Work out the finished part from the listing and answer in its coordinate system (mm). Face numbers are marked on the shaded views. A direction names the side the tool comes from. Give positions to 0.01 mm unless a question says otherwise; leave off trailing zeros. Loops run counter-clockwise (first coordinate to the right, second up) from the corner with the lowest first, then second, coordinate; pieces in that order, holes last. Notation, with made-up numbers: M -24,77.25 L 25,77.25 A23 cw 25,97.25 Z; hole C 72.5,45 d4. An arc over 180 degrees is marked long. Use a Markdown table: item, result.
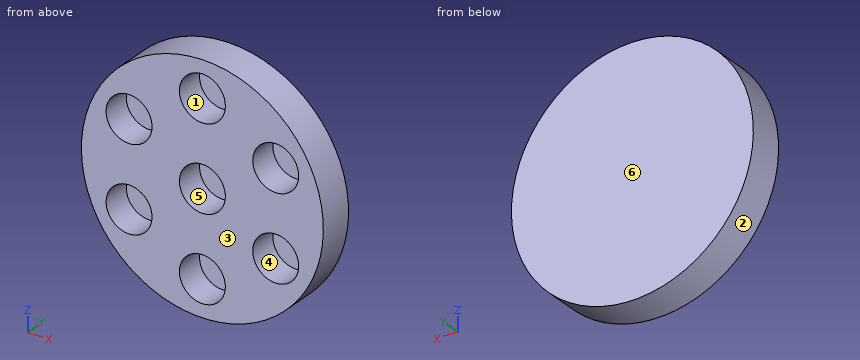
```python
from build123d import *

# Parameters (mm, degrees)
SKETCH1_R           = 25.4
BOSS_EXTRUDE2_DEPTH = 7.62
SKETCH4_R           = 4.826
CUT_EXTRUDE2_DEPTH  = 6.096
CIRPATTERN1_COUNT   = 6
SKETCH5_R           = 4.826
CUT_EXTRUDE6_DEPTH  = 6.096
SCALE1_SCALE        = 0.5


with BuildPart() as part:
    # Sketch1 → Boss-Extrude2 (new body)
    with BuildSketch(Plane(origin=(0, 0, 0), x_dir=(1, 0, 0), z_dir=(0, 1, 0))):
        with Locations(Location((0, 0, 0), (0, 0, 270))):
            Circle(SKETCH1_R)
    extrude(amount=BOSS_EXTRUDE2_DEPTH)

    # Sketch4 → Cut-Extrude2 (cut)
    with BuildSketch(Plane(origin=(0, 0, 0), x_dir=(1, 0, 0), z_dir=(0, 1, 0))):
        with Locations(Location((0, 17.78, 0), (0, 0, 90))):
            Circle(SKETCH4_R)
    cut_extrude2 = extrude(amount=CUT_EXTRUDE2_DEPTH, mode=Mode.SUBTRACT)

    # CirPattern1: Cut-Extrude2 ×6 about axis
    cirpattern1_axis = Axis((0, 0, 0), (0, 1, 0))
    for i in range(1, CIRPATTERN1_COUNT):
        add(cut_extrude2.rotate(cirpattern1_axis, i * 360 / CIRPATTERN1_COUNT), mode=Mode.SUBTRACT)

    # Sketch5 → Cut-Extrude6 (cut)
    with BuildSketch(Plane(origin=(0, 0, 0), x_dir=(1, 0, 0), z_dir=(0, 1, 0))):
        with Locations(Location((0, 0, 0), (0, 0, 90))):
            Circle(SKETCH5_R)
    extrude(amount=CUT_EXTRUDE6_DEPTH, mode=Mode.SUBTRACT)


with BuildPart() as part_1:
    # Scale1: scaled about (0, 4.003078713, 0)
    add(part.part.scale(SCALE1_SCALE).moved(Location((0, 2.001539356, 0))))


solid = part_1.part
```
(1) A cutting plane is placed at D-D (z = -8.89). Write down the section's boundary in (x, y).
Entries:
| item | result |
|---|---|
| outline | M -9.07,2 L -2.41,2 L -2.41,5.05 L 2.41,5.05 L 2.41,2 L 9.07,2 L 9.07,5.81 L -9.07,5.81 Z |
(2) Consider probe 1 along X at (y, z) = (4, -4.25); probe 2 along X at (y, z) = (4.6, 3.5); probe 3 along Y at (x, z) = (1.25, 7.25). Determine where each line is inside the solid, lowest interval first. Write a range as [from, to].
Entries:
| item | result |
|---|---|
| probe 1 | x = [-11.97, -10.1], [-5.29, 5.29], [10.1, 11.97] |
| probe 2 | x = [-12.21, -9.92], [-5.48, 5.48], [9.92, 12.21] |
| probe 3 | y = [5.05, 5.81] |
(3) The mould has two halves that part along Z. Classify the marked faces 1, 2, 3 and 4: released by +Z, released by -Z, zero draft, split by the parting line, or undercut.
Entries:
| item | result |
|---|---|
| face 1 | undercut |
| face 2 | split by the parting line |
| face 3 | zero draft |
| face 4 | undercut |
(4) Which of the six approach directions +Z, -Z, +X, -X, +Y, -Y give full straight-line access (tool end or side, diameter ignored) to the marked faces 5 and 6?
Entries:
| item | result |
|---|---|
| face 5 | -Y |
| face 6 | +Z, -Z, +X, -X, +Y |
(5) A cutting plane is placed at A-A (x = 0). Write down the section's boundary in (y, z), and give its area (3 significant figures).
Entries:
| item | result |
|---|---|
| outline | M 2,-12.7 L 5.81,-12.7 L 5.81,12.7 L 2,12.7 L 2,11.3 L 5.05,11.3 L 5.05,6.48 L 2,6.48 L 2,2.41 L 5.05,2.41 L 5.05,-2.41 L 2,-2.41 L 2,-6.48 L 5.05,-6.48 L 5.05,-11.3 L 2,-11.3 Z |
| area | 52.6 mm² |
(6) A cutting plane is placed at C-C (y = 2.7). Write down the section's boundary in (x, z) (1 decimal), and give its area (3 significant figures).
Entries:
| item | result |
|---|---|
| outline | C 0,0 d25.4; hole C -7.7,-4.4 d4.8; hole C -7.7,4.4 d4.8; hole C 0,-8.9 d4.8; hole C 0,0 d4.8; hole C 0,8.9 d4.8; hole C 7.7,-4.4 d4.8; hole C 7.7,4.4 d4.8 |
| area | 379 mm² |
(7) A cutting plane is placed at B-B (z = 0). Write down the section's boundary in (x, y).
Entries:
| item | result |
|---|---|
| outline | M -12.7,2 L -2.41,2 L -2.41,5.05 L 2.41,5.05 L 2.41,2 L 12.7,2 L 12.7,5.81 L -12.7,5.81 Z |
(8) Given P1, Ø1.5, axis at y = 3, z = -6, coming from the -X side; P2, Ø1, axis at y = 4.5, z = -1.5, coming from the +X side; P3, Ø1.5, axis at y = 5, z = 2.5, coming from the +X side, each flat-ended and moving along its own axis, determine where each tip first touches the part or whether it passes through.
Entries:
| item | result |
|---|---|
| P1 | stops at x = -11.56 |
| P2 | stops at x = 12.66 |
| P3 | stops at x = 12.58 |
